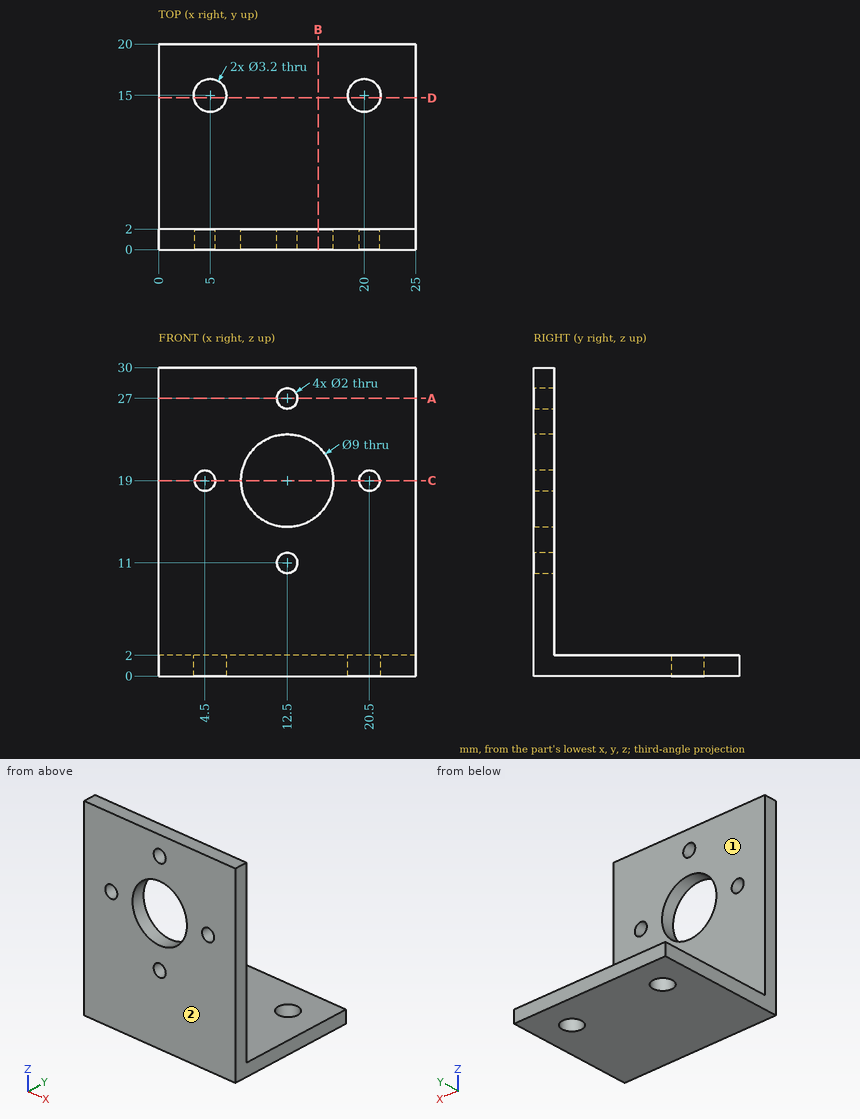
Source: three-view drawing plus pictorial views. Frame: mm from the lowest corner of the part. A direction names the side the tool comes from. Round coordinates to 2 decimals unless told otherwise and drop trailing zeros. Order: outer loops, then holes, each group sorted by start corner. A loop starts at its lowest first (then second) coordinate and runs counter-clockwise, first axis right, second up. Notation, with made-up numbers: (78.25, 30.5) -> (84.25, 30.5) arc R11 cw to (84.25, 34.5) -> close; hole circle Ø10 at (-35.5, 74). An arc over 180 degrees is marked (long way). Use one line per item in the form item = value.
(1) Section C-C on z = 19. Return loops of the section in (x, y), and give its area (3 significant figures).
Results list:
outline = (0, 0) -> (3.5, 0) -> (3.5, 2) -> (0, 2) -> close; (5.5, 0) -> (8, 0) -> (8, 2) -> (5.5, 2) -> close; (17, 0) -> (19.5, 0) -> (19.5, 2) -> (17, 2) -> close; (21.5, 0) -> (25, 0) -> (25, 2) -> (21.5, 2) -> close
area = 24.0 mm^2
(2) Ray query, probe 1 along X at (y, z) = (1.2, 19); probe 2 along Z at (x, y) = (12.5, 1.55); probe 3 along X at (y, z) = (0.6, 11). Return the intervals inside material, ascending. Write a range as [from, to].
Results list:
probe_1 = [0, 3.5], [5.5, 8], [17, 19.5], [21.5, 25]
probe_2 = [0, 10], [12, 14.5], [23.5, 26], [28, 30]
probe_3 = [0, 11.5], [13.5, 25]
(3) Section A-A on z = 27. Return loops of the section in (x, y).
Results list:
outline = (0, 0) -> (11.5, 0) -> (11.5, 2) -> (0, 2) -> close; (13.5, 0) -> (25, 0) -> (25, 2) -> (13.5, 2) -> close
(4) Section D-D on y = 14.75. Return loops of the section in (x, z).
Results list:
outline = (0, 0) -> (3.42, 0) -> (3.42, 2) -> (0, 2) -> close; (6.58, 0) -> (18.42, 0) -> (18.42, 2) -> (6.58, 2) -> close; (21.58, 0) -> (25, 0) -> (25, 2) -> (21.58, 2) -> close
(5) Section B-B on x = 15.5. Return loops of the section in (y, z).
Results list:
outline = (0, 0) -> (20, 0) -> (20, 2) -> (2, 2) -> (2, 15.65) -> (0, 15.65) -> close; (0, 22.35) -> (2, 22.35) -> (2, 30) -> (0, 30) -> close
(6) First-contact query: pin 1 Ø7.5 at (x, z) = (16, 14.5) entering from +Y; pin 2 Ø1.8 at (x, z) = (12.5, 11) entering from -Y; pin 3 Ø4 at (x, y) = (5, 15) entering from +Z. Flat tips, straight axial feed; report the tip coordinate or a pass-through.
Results list:
pin_1 = 2
pin_2 = through
pin_3 = 2
(7) Access query for the marked faces 1 and 2. Directions: +Z, -Z, +X, -X, +Y, -Y. A direction counts if a zero-diameter tool reaches every point of the face in a straight line with its end or side. Return the directions, or none.
Results list:
face_1 = +Z, +X, -X, +Y
face_2 = +Z, -Z, +X, -X, -Y
